```python
from build123d import *

# Parameters (mm, degrees)
BOSS_EXTRUDE1_DEPTH = 5
FILLET1_R           = 5
FILLET2_R           = 1


with BuildPart() as part:
    # Sketch1 → Boss-Extrude1 (new body)
    with BuildSketch(Plane.XY):
        Polygon((215, 55.05), (215, 60), (132.5, 60), (107.5, 85), (82.5, 60), (0, 60), (0, 55.05), (-5, 55.05), (-5, 14.95), (0, 14.95), (0, 0), (215, 0), (215, 14.95), (220, 14.95), (220, 55.05), align=None)
    extrude(amount=BOSS_EXTRUDE1_DEPTH)

    # Fillet1
    fillet1_edges = [part.edges().sort_by_distance(p)[0] for p in [
        (82.5, 60, 2.5),
        (107.5, 85, 2.5),
        (132.5, 60, 2.5),
    ]]
    fillet(fillet1_edges, radius=FILLET1_R)

    # Fillet2
    fillet2_edges = [part.edges().sort_by_distance(p)[0] for p in [
        (-5, 14.95, 2.5),
        (-5, 55.05, 2.5),
        (220, 55.05, 2.5),
        (220, 14.95, 2.5),
    ]]
    fillet(fillet2_edges, radius=FILLET2_R)


solid = part.part
```
Part model, mm, in its own coordinate system. A direction names the side the tool comes from. Round coordinates to 2 decimals unless told otherwise and drop trailing zeros. Loops run counter-clockwise (first coordinate to the right, second up) from the corner with the lowest first, then second, coordinate; pieces in that order, holes last. Notation, with made-up numbers: (74.25, 27.25) -> (108.25, 27.25) arc R20 cw to (108.25, 39.25) -> close; hole circle Ø6 at (88, 59). An arc over 180 degrees is marked (long way). Use a Markdown table: item, result.
1) Cut at A-A, the plane z = 4. List the corners of the cut face in (x, y).
The answers:
| item | result |
|---|---|
| outline | (-5, 15.95) arc R1 ccw to (-4, 14.95) -> (0, 14.95) -> (0, 0) -> (215, 0) -> (215, 14.95) -> (219, 14.95) arc R1 ccw to (220, 15.95) -> (220, 54.05) arc R1 ccw to (219, 55.05) -> (215, 55.05) -> (215, 60) -> (134.57, 60) arc R5 cw to (131.04, 61.46) -> (111.04, 81.46) arc R5 ccw to (103.96, 81.46) -> (83.96, 61.46) arc R5 cw to (80.43, 60) -> (0, 60) -> (0, 55.05) -> (-4, 55.05) arc R1 ccw to (-5, 54.05) -> close |
2) Drop flat-ended pins along their axis: pin 1 Ø1.2 at (x, z) = (-1, 3) entering from +Y; pin 2 Ø1.5 at (x, z) = (33.5, 1.5) entering from +Y; pin 3 Ø2.5 at (y, z) = (58, 3) entering from -X. Give the stop position or say it passes through.
The answers:
| item | result |
|---|---|
| pin 1 | stops at y = 55.05 |
| pin 2 | stops at y = 60 |
| pin 3 | stops at x = 0 |
3) Cut at B-B, the plane y = 77. List the corners of the cut face in (x, z).
The answers:
| item | result |
|---|---|
| outline | (99.5, 0) -> (115.5, 0) -> (115.5, 5) -> (99.5, 5) -> close |
4) Probe line 1 (Y direction, x = 63.5, z = 2.7); line 2 (X direction, y = 14, z = 4.6); line 3 (X direction, y = 76, z = 3.5). List the from-to ranges inside material, lowest first. Write a range as [from, to].
The answers:
| item | result |
|---|---|
| line 1 | y = [0, 60] |
| line 2 | x = [0, 215] |
| line 3 | x = [98.5, 116.5] |
5) Tool access for faces 1 (the flat face through (217, 55.05, 2)), 2 (the flat face through (41, 60, 2)), 3 (the flat face through (217, 14.95, 2)), 4 (the flat face through (220, 35, 2)), 5 (the flat face through (0, 8, 2)): list every direction of +Z, -Z, +X, -X, +Y, -Y with a clear straight run to the whole face (end or side of a thin tool).
The answers:
| item | result |
|---|---|
| face 1 | +Z, -Z, +X, +Y |
| face 2 | +Z, -Z, -X, +Y |
| face 3 | +Z, -Z, +X, -Y |
| face 4 | +Z, -Z, +X, +Y, -Y |
| face 5 | +Z, -Z, -X, -Y |
6) Cut at C-C, the plane x = 143.5. List the corners of the cut face in (y, z), and give its area (3 significant figures).
The answers:
| item | result |
|---|---|
| outline | (0, 0) -> (60, 0) -> (60, 5) -> (0, 5) -> close |
| area | 300 mm2 |
